Geometry: final body of the model. Coordinates: model frame, mm. A direction names the side the tool comes from. Give positions to 0.01 mm unless a question says otherwise; leave off trailing zeros. Loops run counter-clockwise (first coordinate to the right, second up) from the corner with the lowest first, then second, coordinate; pieces in that order, holes last. Notation, with made-up numbers: (62, 13) -> (89, 13) arc R28 ccw to (89, 38) -> close; hole circle Ø3 at (47, 66). An arc over 180 degrees is marked (long way). Answer in a Markdown table with one row per item. Add a question column.
1) Access query for faces 1 (the conical face through (21.863, -3.254, -27.077)), 2 (the flat face through (52, -6, -11.517)). Directions: +Z, -Z, +X, -X, +Y, -Y. A direction counts if a zero-diameter tool reaches every point of the face in a straight line with its end or side. Return the directions, or none.
2) Section query C-C (z = -45). Return the cut outline in (x, y), plus the area to 3 significant figures.
3) Section query D-D (x = 50.5). Return the cut outline in (y, z).
4) First-contact query: P1, Ø6.5, axis at x = 49.5, y = -6.5, coming from the +Z side; P2, Ø4, axis at x = 60, z = -15, coming from the +Y side; P3, Ø8.5, axis at x = 20, z = -30, coming from the +Y side. Flat tips, straight axial feed; report the tip coordinate or a pass-through.
5) Section query B-B (y = -10.75). Return the cut outline in (x, z).
6) Draft query along X for faces 3 (the cylindrical face through (63.5, -6.6, -45.1)), 4 (the flat face through (0, -6, -30)), 5 (the flat face through (75, -6, -30)), 6 (the flat face through (37, -13, -30)). Return one class per face: +X half, -X half, draft (parallel to the pull), parting line (faces both ways), or undercut.
7) Section query A-A (x = 20). Return the cut outline in (y, z).
8) Line query: line 1 (Z direction, x = 51.5, y = -8.75); line 2 (X direction, y = -3, z = -15); line 3 (X direction, y = -5.25, z = -30). Output: solid intervals per line, ascending. Write a range as from..to.
```python
from build123d import *

# Parameters (mm, degrees)
F0_W           = 75
F0_H           = 60
F1_DEPTH       = 13
F3_D           = 6.6
F3_CSINK_D     = 13.44
F3_CSINK_ANGLE = 90
F5_D           = 7
F7_DEPTH       = 25
F9_DEPTH       = 25


with BuildPart() as f1:
    # F0 (on Front) → F1 (new body)
    with BuildSketch(Plane.XZ):
        with Locations((37.5, -30)):
            Rectangle(F0_W, F0_H)
    extrude(amount=F1_DEPTH)

    # F3 (through all)
    with Locations(Plane(origin=(0, 0, 0), x_dir=(-1, 0, 0), z_dir=(0, 1, 0))):
        with Locations((-20, -30)):
            CounterSinkHole(F3_D / 2, F3_CSINK_D / 2, counter_sink_angle=F3_CSINK_ANGLE)

    # F5 (through all)
    with Locations(Plane(origin=(0, 0, 0), x_dir=(-1, 0, 0), z_dir=(0, 1, 0))):
        with Locations((-45, -45), (-60, -45), (-60, -15), (-45, -15)):
            Hole(F5_D / 2)

    # F6 (on face) → F7 (cut)
    with BuildSketch(Plane(origin=(0, 0, 0), x_dir=(-1, 0, 0), z_dir=(0, 1, 0))):
        Polygon((-59.9996023931, -48.4999999774), (-45.1088056195, -48.4983083536), (-45.0000000053, -41.5), (-59.9996023931, -41.5000000226), align=None)
    extrude(amount=-F7_DEPTH, mode=Mode.SUBTRACT)

    # F8 (on face) → F9 (cut)
    with BuildSketch(Plane(origin=(0, 0, 0), x_dir=(-1, 0, 0), z_dir=(0, 1, 0))):
        with BuildLine():
            Line((-45.3417231841, -11.5167220517), (-59.6582768159, -11.5167220517))
            ThreePointArc((-59.6582768159, -11.5167220517), (-57.4071221448, -12.64904606), (-56.5, -15))
            ThreePointArc((-56.5, -15), (-57.4071221448, -17.35095394), (-59.6582768159, -18.4832779483))
            Line((-59.6582768159, -18.4832779483), (-45.3417231841, -18.4832779483))
            ThreePointArc((-45.3417231841, -18.4832779483), (-48.5, -15), (-45.3417231841, -11.5167220517))
        make_face()
    extrude(amount=-F9_DEPTH, mode=Mode.SUBTRACT)


solid = f1.part
```
Evaluation:
| question | item | result |
|---|---|---|
| 1 | face 1 | +Y |
| 1 | face 2 | +Y, -Y |
| 2 | outline | (0, -13) -> (41.5, -13) -> (41.5, 0) -> (0, 0) -> close; (63.5, -13) -> (75, -13) -> (75, 0) -> (63.5, 0) -> close |
| 2 | area | 689 mm² |
| 3 | outline | (-13, -60) -> (0, -60) -> (0, -48.5) -> (-13, -48.5) -> close; (-13, -41.5) -> (0, -41.5) -> (0, -18.48) -> (-13, -18.48) -> close; (-13, -11.52) -> (0, -11.52) -> (0, 0) -> (-13, 0) -> close |
| 4 | P1 | z = 0 |
| 4 | P2 | through |
| 4 | P3 | y = -2.47 |
| 5 | outline | (0, -60) -> (75, -60) -> (75, 0) -> (0, 0) -> close; hole circle Ø6.6 at (20, -30); hole (45, -41.5) arc R3.5 ccw (long way) to (45.11, -48.5) -> (60, -48.5) arc R3.5 ccw to (60, -41.5) -> close; hole (45.34, -18.48) -> (59.66, -18.48) arc R3.5 ccw (long way) to (59.66, -11.52) -> (45.34, -11.52) arc R3.5 ccw (long way) to start |
| 6 | face 3 | undercut |
| 6 | face 4 | -X half |
| 6 | face 5 | +X half |
| 6 | face 6 | draft |
| 7 | outline | (-13, -60) -> (0, -60) -> (0, -36.72) -> (-3.42, -33.3) -> (-13, -33.3) -> close; (-13, -26.7) -> (-3.42, -26.7) -> (0, -23.28) -> (0, 0) -> (-13, 0) -> close |
| 8 | line 1 | -60..-48.5, -41.5..-18.48, -11.52..0 |
| 8 | line 2 | 0..41.5, 63.5..75 |
| 8 | line 3 | 0..16.7, 23.3..75 |
